Can you work these out from the drawing? Everything is in mm from the part's minimum corner. A direction names the side the tool comes from. Coordinates: 2 decimals unless noted, no trailing zeros. Order: outer loops, then holes, each group sorted by start corner. A loop starts at its lowest first (then second) coordinate and runs counter-clockwise, first axis right, second up. Notation, with made-up numbers: (14, 0) -> (37, 0) arc R14 ccw to (37, 21) -> close; hole circle Ø4 at (-12.5, 56). An arc over 180 degrees is marked (long way). Use a Markdown table: item, result. Add a question column.
1) If we section it at A-A (y = 30.5): Write out the boundary of the cut face in (x, z).
2) If I drill on L1, parallel to Z at x = 53, y = 46.5, over which ranges is the centre line in solid material (lowest first)? Write a range as [from, to].
3) If we section it at B-B (x = 20): Write out the boundary of the cut face in (y, z).
4) Will these pins go through, and if not, where does the flat tip stop? pin 1 Ø1 at (x, z) = (26, 85) entering from +Y; pin 2 Ø4 at (y, z) = (9, 75) entering from -X; pin 3 Ø2 at (x, y) = (20, 17.5) entering from +Z.
5) Which directions (+Z, -Z, +X, -X, +Y, -Y) give clear straight access to the entire face, cutting with the end or side of a thin tool? Please do the marked faces 1 and 2.
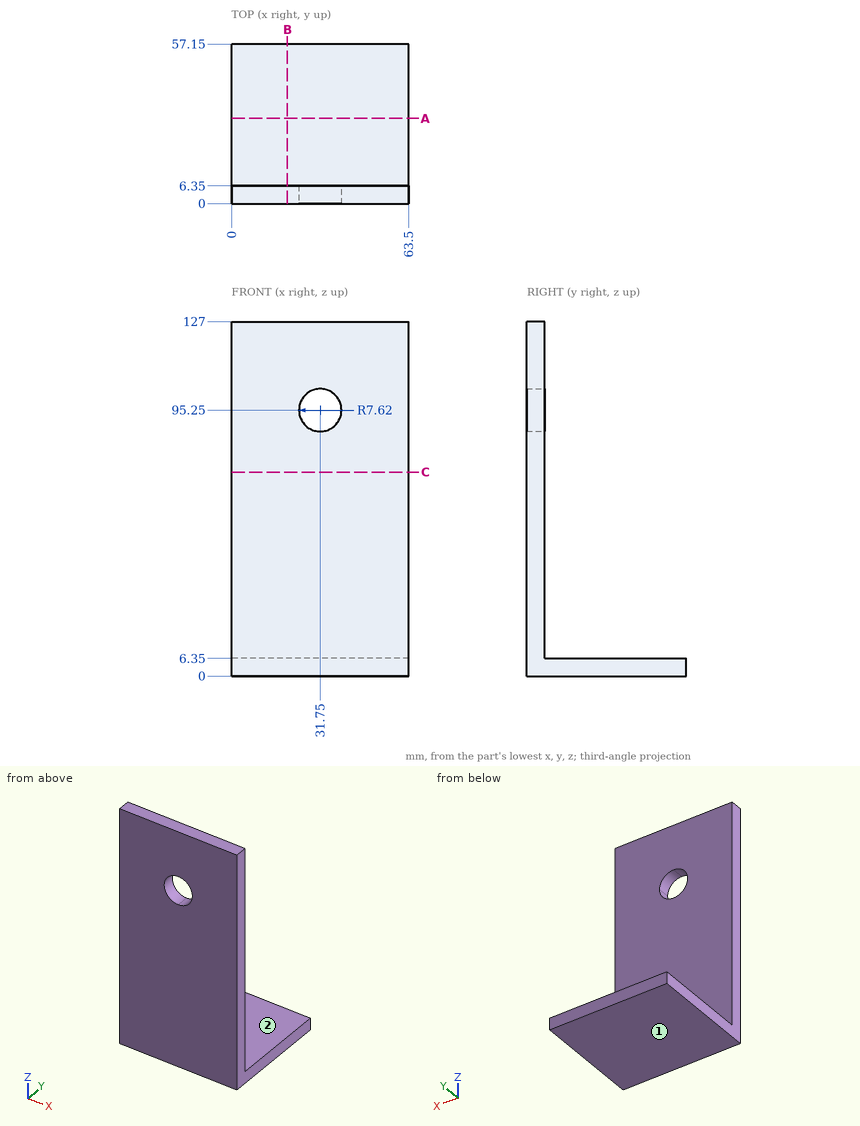
Answer sheet:
| question | item | result |
|---|---|---|
| 1 | outline | (0, 0) -> (63.5, 0) -> (63.5, 6.35) -> (0, 6.35) -> close |
| 2 | L1 | [0, 6.35] |
| 3 | outline | (0, 0) -> (57.15, 0) -> (57.15, 6.35) -> (6.35, 6.35) -> (6.35, 127) -> (0, 127) -> close |
| 4 | pin 1 | y = 6.35 |
| 4 | pin 2 | through |
| 4 | pin 3 | z = 6.35 |
| 5 | face 1 | -Z, +X, -X, +Y, -Y |
| 5 | face 2 | +Z, +X, -X, +Y |
